```python
from build123d import *

# Parameters (mm, degrees)
SKETCH_1_R               = 2
EXTRUDE_1_DEPTH          = 2.6
SKETCH_2_R               = 2.9
EXTRUDE_2_DEPTH          = 1
CUT_EXTRUDE_1_DEPTH      = 6.45710546
CUT_EXTRUDE_1_DEPTH_BACK = 6.45710546
SKETCH_3_R               = 0.8
FILLET_2_R               = 0.5


with BuildPart() as part:
    # 草图1 → 凸台-拉伸1 (new body)
    with BuildSketch(Plane.XY):
        Circle(SKETCH_1_R)
    extrude(amount=EXTRUDE_1_DEPTH)

    # 草图2 → 凸台-拉伸2 (add)
    with BuildSketch(Plane.XY.offset(2.6)):
        Circle(SKETCH_2_R)
    extrude(amount=EXTRUDE_2_DEPTH)

    # 草图3 → 切除-拉伸1 (cut, two sides: drawn at the far end of the back side and taken through both)
    with BuildSketch(Plane.XY.offset(3.6).offset(-CUT_EXTRUDE_1_DEPTH_BACK)):
        Circle(SKETCH_3_R)
    extrude(amount=CUT_EXTRUDE_1_DEPTH + CUT_EXTRUDE_1_DEPTH_BACK, mode=Mode.SUBTRACT)

    # 圆角2
    fillet_2_edges = [part.edges().sort_by_distance(p)[0] for p in [
        (-2, 0, 0),
        (-2.9, 0, 2.6),
        (-2.9, 0, 3.6),
    ]]
    fillet(fillet_2_edges, radius=FILLET_2_R - 0.0001)  # a hair under: the kernel refuses the full size


solid = part.part
```
Read the model definition and answer for the solid it produces. Units are mm, in the model's axes. A direction names the side the tool comes from. Give positions to 0.01 mm unless a question says otherwise; leave off trailing zeros. Loops run counter-clockwise (first coordinate to the right, second up) from the corner with the lowest first, then second, coordinate; pieces in that order, holes last.
Item 1: Find the intervals of material crossed by line 1 along Y through (x, z) = (0, 1.9); line 2 along Z through (x, y) = (0.15, -2.5); line 3 along X through (y, z) = (-0.2, 2.45), in increasing order.
Item 2: Each of these flat-tipped pins is pushed along its axis until it touches: pin 1 Ø1.5 at (x, z) = (0.5, 1.5) entering from +Y; pin 2 Ø1 at (x, y) = (0, 0) entering from +Z; pin 3 Ø1 at (x, z) = (2, 3) entering from -Y; pin 4 Ø1 at (x, z) = (-2, 2.5) entering from +Y. Where does it stop, or does it pass through?
Item 3: For faces 1 (the flat face through (-1, 2, 2.6)), 2 (the flat face through (1, 0, 0)), determine the directions among +Z, -Z, +X, -X, +Y, -Y from which every point of the face is accessible in a straight line to the end or side of a thin tool.
Item 4: The part is cut by section C-C (z = 1.6). Write down the section's boundary in (x, y), and give its area (3 significant figures).
Item 5: The mould has two halves that part along X. Classify faces 3 (the cylindrical face through (0, -2, 2)), 4 (the cylindrical face through (-0.63, -0.49, 1.77)), 5 (the flat face through (-1, 1, 3.6)): released by +X, released by -X, zero draft, split by the parting line, or undercut.
Taken from the geometry:
1. line 1: y = -2 to -0.8, 0.8 to 2
1. line 2: z = 2.61 to 3.59
1. line 3: x = -1.99 to -0.77, 0.77 to 1.99
2. pin 1: stops at y = 2
2. pin 2: passes through
2. pin 3: stops at y = -2.48
2. pin 4: stops at y = 2.31
3. face 1: -Z
3. face 2: -Z, +X, -X, +Y, -Y
4. outline: circle Ø4 at (0, 0); hole circle Ø1.6 at (0, 0)
4. area: 10.6 mm2
5. face 3: split by the parting line
5. face 4: undercut
5. face 5: zero draft
